The model under review builds one solid part; all positions refer to its coordinate system, in mm. Face numbers are marked on the shaded views. A direction names the side the tool comes from. Round coordinates to 2 decimals unless told otherwise and drop trailing zeros. Write each loop counter-clockwise with the first axis right and the second up, starting at its lowest first coordinate (ties: lowest second). Pieces come first, ordered by that corner, then holes. Notation, with made-up numbers: (-2, -36) - (16, -36) arc R11 ccw to (16, -24) - close; hole circle Ø6 at (-4.5, -16.75). An arc over 180 degrees is marked (long way). Use one line per item in the form item = value.
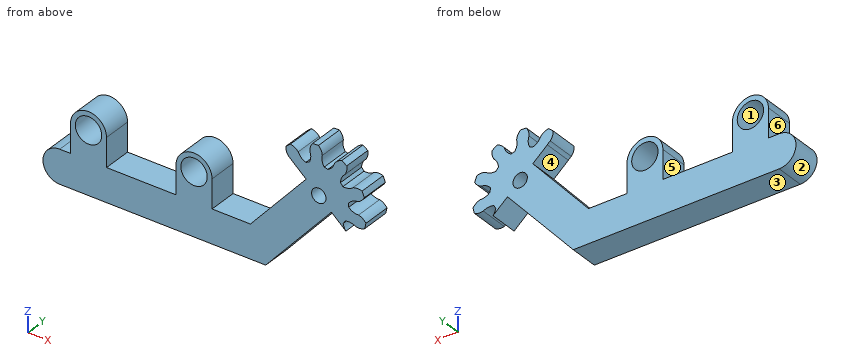
from build123d import *

# Parameters (mm, degrees)
CROQUIS1_R              = 2.75
SALIENTE_EXTRUIR1_DEPTH = 6
CROQUIS2_R              = 1.5
CORTAR_EXTRUIR1_DEPTH   = 62.68062905
SALIENTE_EXTRUIR2_START = -6
SALIENTE_EXTRUIR2_DEPTH = 6
CORTAR_EXTRUIR2_DEPTH   = 71.114192572


with BuildPart() as part:
    # Croquis1 → Saliente-Extruir1 (new body)
    with BuildSketch(Plane(origin=(0, 0, 0), x_dir=(1, 0, 0), z_dir=(0, 1, 0))):
        with BuildLine():
            Line((42.930999161, 0), (56.636539912, -15.69811875))
            ThreePointArc((56.636539912, -15.69811875), (56.30188125, -20.636539912), (51.363460088, -20.30188125))
            Line((51.363460088, -20.30188125), (39.75, -7))
            Line((39.75, -7), (31.75, -7))
            Line((31.75, -7), (31.75, -13))
            ThreePointArc((31.75, -13), (28, -16.75), (24.25, -13))
            Line((24.25, -13), (24.25, -7))
            Line((24.25, -7), (9.75, -7))
            Line((9.75, -7), (9.75, -13))
            ThreePointArc((9.75, -13), (6, -16.75), (2.25, -13))
            Line((2.25, -13), (2.25, -7))
            Line((2.25, -7), (0, -7))
            ThreePointArc((0, -7), (-3.5, -3.5), (0, 0))
            Line((0, 0), (42.930999161, 0))
        make_face()
        with Locations(Location((28, -13, 0), (0, 0, 270))):
            Circle(CROQUIS1_R, mode=Mode.SUBTRACT)
        with Locations(Location((6, -13, 0), (0, 0, 270))):
            Circle(CROQUIS1_R, mode=Mode.SUBTRACT)
    extrude(amount=SALIENTE_EXTRUIR1_DEPTH)

    # Croquis2 → Cortar-Extruir1 (cut, through all)
    with BuildSketch(Plane(origin=(0, 6, 0), x_dir=(1, 0, 0), z_dir=(0, 1, 0))):
        with Locations(Location((54, -18, 0), (0, 0, 270))):
            Circle(CROQUIS2_R)
    extrude(amount=-CORTAR_EXTRUIR1_DEPTH, mode=Mode.SUBTRACT)

    # Croquis3 → Saliente-Extruir2 (add)
    with BuildSketch(Plane(origin=(0, 6, 0), x_dir=(1, 0, 0), z_dir=(0, 1, 0)).offset(SALIENTE_EXTRUIR2_START)):
        with BuildLine():
            Line((51.363460088, -20.30188125), (46.467028822, -24.576803572))
            ThreePointArc((46.467028822, -24.576803572), (60.576803572, -25.532971178), (61.532971178, -11.423196428))
            Line((61.532971178, -11.423196428), (56.636539912, -15.69811875))
            ThreePointArc((56.636539912, -15.69811875), (56.30188125, -20.636539912), (51.363460088, -20.30188125))
        make_face()
    extrude(amount=SALIENTE_EXTRUIR2_DEPTH)

    # Croquis4 → Cortar-Extruir2 (cut, through all)
    with BuildSketch(Plane(origin=(0, 6, 0), x_dir=(1, 0, 0), z_dir=(0, 1, 0))):
        with BuildLine():
            ThreePointArc((44.471919223, -21.035733308), (45.527460474, -23.311880456), (47.116349204, -25.25364403))
            ThreePointArc((47.116349204, -25.25364403), (47.255351375, -24.311140987), (47.722398468, -23.480779257))
            ThreePointArc((47.722398468, -23.480779257), (48.523826653, -22.694010434), (48.921868449, -21.643841379))
            ThreePointArc((48.921868449, -21.643841379), (48.704493345, -21.320031523), (48.507736999, -20.983294683))
            ThreePointArc((48.507736999, -20.983294683), (47.389059112, -20.884036937), (46.331721606, -21.262626046))
            ThreePointArc((46.331721606, -21.262626046), (45.380828681, -21.321245459), (44.471919223, -21.035733308))
        make_face()
        with BuildLine():
            ThreePointArc((48.075979996, -26.056425199), (50.267816532, -27.277435344), (52.694594509, -27.914429711))
            ThreePointArc((52.694594509, -27.914429711), (52.253060238, -27.070225306), (52.142834895, -26.123925161))
            ThreePointArc((52.142834895, -26.123925161), (52.328752805, -25.016348145), (52.0335015, -23.932780435))
            ThreePointArc((52.0335015, -23.932780435), (51.667310689, -23.798582639), (51.310202513, -23.641807292))
            ThreePointArc((51.310202513, -23.641807292), (50.346830851, -24.219048452), (49.713955935, -25.146820868))
            ThreePointArc((49.713955935, -25.146820868), (48.979123025, -25.753165807), (48.075979996, -26.056425199))
        make_face()
        with BuildLine():
            ThreePointArc((53.94281506, -27.999836493), (56.433739822, -27.699325259), (58.771460342, -26.788240222))
            ThreePointArc((58.771460342, -26.788240222), (57.918040714, -26.364791844), (57.272645269, -25.664007776))
            ThreePointArc((57.272645269, -25.664007776), (56.772038582, -24.658679342), (55.896270139, -23.955599013))
            ThreePointArc((55.896270139, -23.955599013), (55.521136064, -24.062272273), (55.140079244, -24.145341273))
            ThreePointArc((55.140079244, -24.145341273), (54.699989039, -25.178594837), (54.73331342, -26.30117303))
            ThreePointArc((54.73331342, -26.30117303), (54.495221721, -27.223640338), (53.94281506, -27.999836493))
        make_face()
        with BuildLine():
            ThreePointArc((59.831492828, -26.123650128), (61.670057221, -24.416402593), (63.025790501, -22.305241669))
            ThreePointArc((63.025790501, -22.305241669), (62.086462807, -22.464292206), (61.152416384, -22.276699911))
            ThreePointArc((61.152416384, -22.276699911), (60.156499839, -21.75762135), (59.034728037, -21.703581191))
            ThreePointArc((59.034728037, -21.703581191), (58.793939164, -22.010379949), (58.534484453, -22.30156376))
            ThreePointArc((58.534484453, -22.30156376), (58.785775205, -23.396161985), (59.472570103, -24.284759241))
            ThreePointArc((59.472570103, -24.284759241), (59.822162551, -25.170997759), (59.831492828, -26.123650128))
        make_face()
        with BuildLine():
            ThreePointArc((63.49273854, -21.144505527), (63.976673456, -18.682632222), (63.832575464, -16.177787128))
            ThreePointArc((63.832575464, -16.177787128), (63.166130956, -16.858584682), (62.300207541, -17.255838039))
            ThreePointArc((62.300207541, -17.255838039), (61.189387409, -17.42127972), (60.250090948, -18.036921234))
            ThreePointArc((60.250090948, -18.036921234), (60.235620444, -18.426658791), (60.196870723, -18.814735096))
            ThreePointArc((60.196870723, -18.814735096), (61.043557906, -19.552578664), (62.121491012, -19.867781033))
            ThreePointArc((62.121491012, -19.867781033), (62.925235175, -20.379277769), (63.49273854, -21.144505527))
        make_face()
        with BuildLine():
            ThreePointArc((63.528080777, -14.964266692), (62.472539526, -12.688119544), (60.883650796, -10.74635597))
            ThreePointArc((60.883650796, -10.74635597), (60.744648625, -11.688859013), (60.277601532, -12.519220743))
            ThreePointArc((60.277601532, -12.519220743), (59.476173347, -13.305989566), (59.078131551, -14.356158621))
            ThreePointArc((59.078131551, -14.356158621), (59.295506655, -14.679968477), (59.492263001, -15.016705317))
            ThreePointArc((59.492263001, -15.016705317), (60.610940888, -15.115963063), (61.668278394, -14.737373954))
            ThreePointArc((61.668278394, -14.737373954), (62.619171319, -14.678754541), (63.528080777, -14.964266692))
        make_face()
    extrude(amount=-CORTAR_EXTRUIR2_DEPTH, mode=Mode.SUBTRACT)


solid = part.part
(1) Add section C-C on z = 3.5. Write out the cut boundary in (x, y).
Geometry results:
outline = (-3.5, 0) - (45.99, 0) - (45.99, 6) - (-3.5, 6) - close
(2) Insertion check: P1, Ø1.5, axis at y = 1.5, z = 19.5, coming from the +X side; P2, Ø3, axis at y = 3, z = 9.5, coming from the -X side; P3, Ø1, axis at y = 5, z = 15.5, coming from the -X side. Each pin has a flat end and moves straight along its axis. Give the tip position at first contact, or say it passes through.
Geometry results:
P1 = 62.78
P2 = 2.25
P3 = 2.83
(3) Add section B-B on y = 3.3. Count the separate pieces of the cut face and the enclosed holes in it, then the cut area to 3 significant figures.
Geometry results:
separate_pieces = 1
enclosed_holes = 3
area = 629 mm2
(4) The part is to be moulded in two halves that separate along X. For the marked faces 1, 2 and 3, say which applies: +X half, -X half, draft (parallel to the pull), parting line (faces both ways), or undercut.
Geometry results:
face_1 = undercut
face_2 = -X half
face_3 = draft
(5) Add section A-A on x = 28. Write out the cut boundary in (y, z).
Geometry results:
outline = (0, 0) - (6, 0) - (6, 10.25) - (0, 10.25) - close; (0, 15.75) - (6, 15.75) - (6, 16.75) - (0, 16.75) - close
(6) To check wall thickness, follow L1, parallel to X at y = 4.7, z = 13; L2, parallel to X at y = 2.2, z = 18; L3, parallel to X at y = 4.35, z = 26.5. State the ranges of each line that lie inside material, in increasing order.
Geometry results:
L1 = 2.25 to 3.25, 8.75 to 9.75, 24.25 to 25.25, 30.75 to 31.75, 44.99 to 54.28
L2 = 49.35 to 52.5, 55.5 to 60.29
L3 = 52.14 to 54.71, 58.12 to 59.27
(7) Machinability: for the marked faces 4, 5 and 6, which of the approach directions +Z, -Z, +X, -X, +Y, -Y give a long, thin tool a straight path to every point of the face, cutting with its end or side? Answer none if there is none.
Geometry results:
face_4 = -X, +Y, -Y
face_5 = +Z, +Y, -Y
face_6 = +Z, -X, +Y, -Y
(8) Add section D-D on x = 41. Write out the cut boundary in (y, z), then the cut area to 3 significant figures.
Geometry results:
outline = (0, 0) - (6, 0) - (6, 8.43) - (0, 8.43) - close
area = 50.6 mm2
